Can you work these out from the model? Positions are in its coordinate system, mm. A direction names the side the tool comes from. Give positions to 0.01 mm unless a question says otherwise; leave off trailing zeros. Loops run counter-clockwise (first coordinate to the right, second up) from the corner with the lowest first, then second, coordinate; pieces in that order, holes last. Notation, with made-up numbers: (44, 55) - (85, 55) arc R24 cw to (85, 66) - close; hole circle Ø2 at (22, -39.5). An arc over 180 degrees is marked (long way). Answer as a JSON object with one key per item and string values.
Autodesk Inventor part; units mm, degrees
ref_plane "YZ Plane" through (0, 0, 0) normal (1, 0, 0) x (0, 1, 0)
ref_plane "XZ Plane" through (0, 0, 0) normal (0, 1, 0) x (-1, 0, 0)
ref_plane "XY Plane" through (0, 0, 0) normal (0, 0, 1) x (1, 0, 0)
sketch "Sketch1" plane through (0, 0, 0) normal (0, 0, 1) x (1, 0, 0)
  line L0 (0, 0) -> (-3.45, 0)
  line L1 (-3.45, 0) -> (-3.45, -20)
  line L2 (-3.45, -20) -> (0, -20)
  line L3 (0, -20) -> (0, 0)
  line L4 (-1.725, -20) -> (-5.425, -20)
  line L5 (-5.425, -20) -> (1.925, -20)
  line L6 (1.925, -20) -> (1.925, -25)
  line L7 (1.925, -25) -> (-5.425, -25)
  line L8 (-5.425, -25) -> (-5.425, -20)
  dimension "d0" = 20
  dimension "d1" = 3.45
  dimension "d2" = 3.7
  dimension "d3" = 7.35
  dimension "d4" = 5
extrude "Extrusion1" add sketch "Sketch1" along normal blind 3.5
sketch "Sketch4" plane through (0, 0, 0) normal (0, 0, -1) x (-1, 0, 0)
  line L0 (0, -20) -> (0, 0)
  line L1 (-1.925, -20) -> (0, -20)
  line L2 (-1.925, -25) -> (-1.925, -20)
  line L3 (5.425, -25) -> (-1.925, -25)
  line L4 (5.425, -20) -> (5.425, -25)
  line L5 (3.45, -20) -> (5.425, -20)
  line L6 (3.45, 0) -> (3.45, -20)
  line L7 (0, 0) -> (3.45, 0)
  line L8 (3.45, 0) -> (5.475, 0)
  line L9 (0, 0) -> (-2.025, 0)
  line L10 (5.475, 0) -> (-2.025, 0)
  line L11 (-2.025, 0) -> (-2.025, 4)
  line L12 (-2.025, 4) -> (5.475, 4)
  line L13 (5.475, 4) -> (5.475, 0)
  circle A0 centre (1.725, 4) radius 3.75
  circle A1 centre (1.725, 4) radius 1.55
  dimension "d22" = 2.025
  dimension "d23" = 2.025
  dimension "d24" = 7.5
  dimension "d25" = 4
  dimension "d26" = 3.1
extrude "Extrusion4" add sketch "Sketch4" against normal up to surface (3.5 mm away) contours L9 L11 A0 L13 L8 L7 | A0 L12 A1 | L12 A1 A0
sketch "Sketch5" plane through (0, 0, 3.5) normal (0, 0, 1) x (1, 0, 0)
  circle A0 centre (-1.725, 4) radius 1.55
  line L0 (0, -20) -> (0, 0)
  line L1 (2.025, 0) -> (0, 0)
  line L2 (2.025, 4) -> (2.025, 0)
  arc A1 (2.025, 4) -> (-5.475, 4) centre (-1.725, 4) ccw
  line L3 (-5.475, 0) -> (-5.475, 4)
  line L4 (-3.45, 0) -> (-5.475, 0)
  line L5 (-3.45, 0) -> (-3.45, -20)
  line L6 (-3.45, -20) -> (-5.425, -20)
  line L7 (-5.425, -20) -> (-5.425, -25)
  line L8 (-5.425, -25) -> (1.925, -25)
  line L9 (1.925, -25) -> (1.925, -20)
  line L10 (1.925, -20) -> (0, -20)
  line L11 (-3.45, -10) -> (0, -10)
  line L12 (-1.725, -10) -> (-1, -10)
  line L13 (-1, -10) -> (-2.45, -10)
  line L14 (-2.45, -10) -> (-2.45, -20)
  line L15 (-2.45, -20) -> (-3.45, -20)
  line L16 (-1, -10) -> (-1, -20)
  line L17 (0, -20) -> (-1, -20)
  dimension "d31" = 1
  dimension "d32" = 1
extrude "Extrusion5" cut sketch "Sketch5" against normal blind 1.75 contours L10 L9 L8 L7 L6 L15 L14 L11 L16 L17
sketch "Sketch6" plane through (0, 0, 1.75) normal (0, 0, 1) x (1, 0, 0)
  line L0 (1.925, -20) -> (1.925, -25)
  line L1 (0, -20) -> (1.925, -20)
  line L2 (-1, -20) -> (0, -20)
  line L3 (-1, -10) -> (-1, -20)
  line L4 (-2.45, -10) -> (-1, -10)
  line L5 (-2.45, -20) -> (-2.45, -10)
  line L6 (-3.45, -20) -> (-2.45, -20)
  line L7 (-5.425, -20) -> (-3.45, -20)
  line L8 (-5.425, -25) -> (-5.425, -20)
  line L9 (1.925, -25) -> (-5.425, -25)
  line L10 (-2.45, -20) -> (-1, -20)
  point P0 (0, 0)
extrude "Extrusion6" cut sketch "Sketch6" against normal up to surface (1.75 mm away) contours L0 L9 L8 L7 L6 L10 L2 L1
sketch "Sketch7" plane through (-1, -20, 3.5) normal (0, -1, 0) x (1, 0, 0)
  line L0 (1, -3.5) -> (1, 0)
  line L1 (0, 0) -> (1, 0)
  line L2 (0, 0) -> (0, -1.75)
  line L3 (-1.45, -1.75) -> (0, -1.75)
  line L4 (-1.45, 0) -> (-1.45, -1.75)
  line L5 (-2.45, 0) -> (-1.45, 0)
  line L6 (-2.45, -3.5) -> (-2.45, 0)
  line L7 (1, -3.5) -> (-2.45, -3.5)
  line L8 (-2.45, -3.5) -> (-2.45, 0)
  line L9 (1, 0) -> (-2.45, 0)
  line L10 (-2.45, -3.5) -> (1, -3.5)
  line L11 (1, -3.5) -> (1, 0)
  line L12 (-1.95, -0.5) -> (-1.95, -3)
  line L13 (-1.95, -3) -> (0.5, -3)
  line L14 (0.5, -3) -> (0.5, -0.5)
  line L15 (0.5, -0.5) -> (-1.95, -0.5)
  point P0 (1, -3.5)
  dimension "d37" = 0.5
extrude "Extrusion7" cut sketch "Sketch7" against normal up to surface (20 mm away) contours L7 L6 L5 L4 L15 L12 L13 L14 L2 L1 L0 | L2 L15 L4 L9
sketch "Sketch8" plane through (-2.45, -20, 1.75) normal (0, -1, 0) x (1, 0, 0)
  line L0 (1.95, 1.25) -> (1.45, 1.25)
  line L1 (1.45, 1.25) -> (1.45, 0)
  line L2 (0, 0) -> (1.45, 0)
  line L3 (0, 1.25) -> (0, 0)
  line L4 (0, 1.25) -> (-0.5, 1.25)
  line L5 (-0.5, 1.25) -> (-0.5, -1.25)
  line L6 (-0.5, -1.25) -> (1.95, -1.25)
  line L7 (1.95, -1.25) -> (1.95, 1.25)
  line L8 (2.45, -1.75) -> (-1, -1.75)
  line L9 (-1, -1.75) -> (-1, 1.75)
  line L10 (-1, 1.75) -> (0.5, 1.75)
  line L11 (0.5, 1.75) -> (0.5, 0.5)
  line L12 (0.5, 0.5) -> (0.95, 0.5)
  line L13 (0.95, 0.5) -> (0.95, 1.75)
  line L14 (0.95, 1.75) -> (2.45, 1.75)
  line L15 (2.45, 1.75) -> (2.45, -1.75)
  line L16 (0, 1.25) -> (0, 1.75)
  line L17 (0, 1.75) -> (-1, 1.75)
  line L18 (-1, 1.75) -> (-1, -1.75)
  line L19 (-1, -1.75) -> (2.45, -1.75)
  line L20 (2.45, -1.75) -> (2.45, 1.75)
  line L21 (2.45, 1.75) -> (1.45, 1.75)
  line L22 (1.45, 0) -> (1.45, 1.75)
  line L23 (0, 0) -> (1.45, 0)
  line L24 (0, 0) -> (0, 1.25)
  point P0 (2.45, -1.75)
extrude "Extrusion8" add sketch "Sketch8" against normal blind 20 contours L0 L22 L14 L15 L8 L9 L10 L16 L4 L5 L6 L7
sketch "Sketch9" plane through (-2.45, 0, 3) normal (0, 0, 1) x (1, 0, 0)
  line L0 (1.45, -10) -> (1.45, 0)
  line L1 (1.45, 0) -> (0, 0)
  line L2 (0, 0) -> (0, -10)
  line L3 (1.45, -10) -> (0, -10)
  line L4 (0, -20) -> (1.45, -20)
  line L5 (1.45, -10) -> (1.45, -20)
  line L6 (0, -10) -> (1.45, -10)
  line L7 (0, -20) -> (0, -10)
  point P0 (2.45, 0)
extrude "Extrusion9" cut sketch "Sketch9" against normal up to surface (3 mm away)
sketch "Sketch11" plane through (0, 0, 3.5) normal (0, 0, 1) x (1, 0, 0)
  line L0 (2.025, 0) -> (0, 0)
  line L1 (2.025, 4) -> (2.025, 0)
  arc A0 (2.025, 4) -> (-5.475, 4) centre (-1.725, 4) ccw
  line L2 (-5.475, 0) -> (-5.475, 4)
  line L3 (-3.45, 0) -> (-5.475, 0)
  line L4 (-3.45, -20) -> (-3.45, 0)
  line L5 (-2.45, -20) -> (-3.45, -20)
  line L6 (-2.45, -20) -> (-2.45, 0)
  line L7 (-1, 0) -> (-2.45, 0)
  line L8 (-1, -20) -> (-1, 0)
  line L9 (0, -20) -> (-1, -20)
  line L10 (0, -20) -> (0, 0)
  circle A1 centre (-1.725, 4) radius 1.55
  line L11 (-1, 0) -> (0, 0)
  line L12 (-2.45, 0) -> (-3.45, 0)
  point P0 (0, 0)
extrude "Extrusion11" cut sketch "Sketch11" against normal blind 1 contours L10 L9 L8 L11 | L6 L5 L4 L12
equation "\"d23\" = d22"
equation "\"d32\" = d31"
properties part number "Piston"
1) Imagine slicing it at C-C on x = 1. Write out the boundary of the cut face in (y, z).
Check sheet entries:
{"outline": "(0, 0) - (6.58, 0) - (6.58, 3.5) - (0, 3.5) - close"}
2) I need wall thicknesses on L1, parallel to X at y = 4, z = 1.45 (3 decimals); L2, parallel to X at y = -8.25, z = 2.3; L3, parallel to Z at x = -3, y = -4.25. Which ranges of each line are inside material? Lowest first, please.
Check sheet entries:
{"L1": "-5.475 to -3.275, -0.175 to 2.025", "L2": "-3.45 to -2.45, -1 to 0", "L3": "0 to 2.5"}
3) Which directions (+Z, -Z, +X, -X, +Y, -Y) give clear straight access to the entire face, cutting with the end or side of a thin tool? Please do faces 4 (the flat face through (-0.5, -9.9, 2.5)), 5 (the flat face through (-3.45, -10, 1)), 6 (the flat face through (-1, -10, 1)), 7 (the flat face through (0, -10, 1)).
Check sheet entries:
{"face 4": "+Z, +X, -X, -Y", "face 5": "+Z, -Z, -X, -Y", "face 6": "+Z, -Z, -Y", "face 7": "+Z, -Z, +X, -Y"}
4) Imagine slicing it at B-B on y = -15. Write out the boundary of the cut face in (x, z).
Check sheet entries:
{"outline": "(-3.45, 0) - (-2.45, 0) - (-2.45, 2.5) - (-3.45, 2.5) - close; (-1, 0) - (0, 0) - (0, 2.5) - (-1, 2.5) - close"}
5) If we mould it in two halves opening along Y, with no side actions, what happens to faces 1 (the flat face through (-0.8, -6.3, 0)), 2 (the cylindrical face through (-3.2, 4.47, 1.73)), 3 (the cylindrical face through (-1.81, 7.75, 1.73))? For each: released by +Y, released by -Y, zero draft, split by the parting line, or undercut.
Check sheet entries:
{"face 1": "zero draft", "face 2": "undercut", "face 3": "released by +Y"}
6) Imagine slicing it at A-A on z = 2. Write out the boundary of the cut face in (x, y) (3 decimals), and give its area (3 significant figures).
Check sheet entries:
{"outline": "(-5.475, 0) - (-3.45, 0) - (-3.45, -20) - (-2.45, -20) - (-2.45, 0) - (-1, 0) - (-1, -20) - (0, -20) - (0, 0) - (2.025, 0) - (2.025, 4) arc R3.75 ccw to (-5.475, 4) - close; hole circle Ø3.1 at (-1.725, 4)", "area": "84.5 mm2"}
7) I'm going to push flat-ended pins straight in: P1, Ø1.2, axis at y = -13, z = 1.5, coming from the -X side; P2, Ø1.2, axis at y = -7, z = 1.5, coming from the +X side; P3, Ø0.5, axis at x = -3, y = -14, coming from the +Z side; P4, Ø3, axis at x = -1.725, y = 4, coming from the -Z side. Where does each tip first touch, or does it pass through?
Check sheet entries:
{"P1": "x = -3.45", "P2": "x = 0", "P3": "z = 2.5", "P4": "through"}
